Can you work these out from the model? Positions are in its coordinate system, mm. A direction names the side the tool comes from. Give positions to 0.01 mm unless a question says otherwise; leave off trailing zeros. Write each loop counter-clockwise with the first axis right and the second up, starting at its lowest first coordinate (ties: lowest second). Pieces come first, ordered by that corner, then holes.
from build123d import *

# Parameters (mm, degrees)
SKETCH002_W     = 400
SKETCH002_H     = 200
PAD001_DEPTH    = 17
SKETCH001_W     = 70
SKETCH001_H     = 60
POCKET_DEPTH    = 17
SKETCH011_W     = 21
SKETCH011_H     = 130
POCKET003_DEPTH = 17.001


with BuildPart() as part:
    # Sketch002 → Pad001 (new body)
    with BuildSketch(Plane.XY):
        Rectangle(SKETCH002_W, SKETCH002_H)
    extrude(amount=PAD001_DEPTH)

    # Sketch001 → Pocket (cut)
    with BuildSketch(Plane.XY):
        with Locations((-130, 0)):
            Rectangle(SKETCH001_W, SKETCH001_H)
    extrude(amount=POCKET_DEPTH, mode=Mode.SUBTRACT)

    # Sketch011 → Pocket003 (cut, through all)
    with BuildSketch(Plane.XY):
        with Locations((-57.925, 0)):
            Rectangle(SKETCH011_W, SKETCH011_H)
    extrude(amount=POCKET003_DEPTH, mode=Mode.SUBTRACT)


with BuildPart() as part_1:
    # Body placement: moved
    add(part.part.moved(Location((0, 0, 185))))


solid = part_1.part
(1) For faces 4 (the face through (-3, 100, 193)), 5 (the face through (-68.425, -1, 193)), which set-ups out of +Z, -Z, +X, -X, +Y, -Y let a thin tool reach every point of the face, with its end or its side?
Returned:
face 4: +Z, -Z, +X, -X, +Y
face 5: +Z, -Z
(2) Imagine slicing it at A-A, the plane y = 50.5. Write out the boundary of the cut face in (x, z) (3 decimals), plus the area to 3 significant figures.
Returned:
outline: (-200, 185) - (-68.425, 185) - (-68.425, 202) - (-200, 202) - close; (-47.425, 185) - (200, 185) - (200, 202) - (-47.425, 202) - close
area: 6,440 mm2
(3) Imagine slicing it at B-B, the plane x = -150.5. Write out the boundary of the cut face in (y, z), plus the area to 3 significant figures.
Returned:
outline: (-100, 185) - (-30, 185) - (-30, 202) - (-100, 202) - close; (30, 185) - (100, 185) - (100, 202) - (30, 202) - close
area: 2,380 mm2
(4) If we mould it in two halves opening along X, with no side actions, what happens to faces 1 (the face through (-200, -1, 193)), 2 (the face through (-3, -100, 193)), 3 (the face through (-58, -65, 193))? For each: +X half, -X half, draft (parallel to the pull), parting line (faces both ways), or undercut.
Returned:
face 1: -X half
face 2: draft
face 3: undercut
(5) Imagine slicing it at D-D, the plane y = 15.5. Write out the boundary of the cut face in (x, z) (3 decimals).
Returned:
outline: (-200, 185) - (-165, 185) - (-165, 202) - (-200, 202) - close; (-95, 185) - (-68.425, 185) - (-68.425, 202) - (-95, 202) - close; (-47.425, 185) - (200, 185) - (200, 202) - (-47.425, 202) - close
(6) Imagine slicing it at C-C, the plane z = 197. Write out the boundary of the cut face in (x, y) (3 decimals).
Returned:
outline: (-200, -100) - (200, -100) - (200, 100) - (-200, 100) - close; hole (-165, -30) - (-95, -30) - (-95, 30) - (-165, 30) - close; hole (-68.425, -65) - (-47.425, -65) - (-47.425, 65) - (-68.425, 65) - close
(7) If I drill on L1, parallel to X at y = -15, z = 186.25 (3 decimals); L2, parallel to Y at x = -158.5, z = 190; L3, parallel to X at y = -32.5, z = 201 (3 decimals), over which ranges is the centre line in solid material (lowest first)?
Returned:
L1: x = -200 to -165, -95 to -68.425, -47.425 to 200
L2: y = -100 to -30, 30 to 100
L3: x = -200 to -68.425, -47.425 to 200
